Input: part model. Units: mm. Frame: model coordinates. Face numbers are marked on the shaded views. A direction names the side the tool comes from. Round coordinates to 2 decimals unless told otherwise and drop trailing zeros. Loops run counter-clockwise (first coordinate to the right, second up) from the corner with the lowest first, then second, coordinate; pieces in that order, holes last. Notation, with made-up numbers: M 19,57 L 27,57 A18 ccw 27,87 Z; hole C 60.5,34.5 d6. An arc over 180 degrees is marked long. Put each result on its own line as item: value. Start each with the question number.
1) Reachability of the marked faces 1 and 2 from +Z, -Z, +X, -X, +Y, -Y: full face, straight path, thin tool, end or side. Return the list, or none.
2) Section B-B on z = -25.5. Output: boundary loops of the cut face in (x, y) (3 decimals).
3) Line query: probe 1 along Y at (x, z) = (0, -151); probe 2 along Y at (x, z) = (0, -106) (3 decimals); probe 3 along Y at (x, z) = (0, -149). Output: solid intervals per line, ascending.
4) Section C-C on x = 0. State how many separate pieces and enclosed holes the cut face has, plus the area to 3 significant figures.
5) Draft query along X for the marked faces 3, 4, 5 and 6. Return one class per face: +X half, -X half, draft (parallel to the pull), parting line (faces both ways), or undercut.
6) Pin query (flat end, axial travel): pin 1 (2 mm diameter, centred on x = 6, z = -95, fed in from +Y); pin 2 (10.5 mm diameter, centred on x = 3.5, y = -2.5, fed in from +Z); pin 3 (16 mm diameter, centred on x = 4, y = 7, fed in from -Z). Return the tip coordinate at first contact, or that it passes through.
7) Section A-A on y = 0. Output: boundary loops of the cut face in (x, z) (3 decimals), plus the area to 3 significant figures.
from build123d import *
from OCP.BRepFilletAPI import BRepFilletAPI_MakeChamfer

# Parameters (mm, degrees)
CHAMFER1_SIZE           = 0.762
CHAMFER1_SIZE2          = 0.876580726
CUT_EXTRUDE1_DEPTH      = 193.922990854
CUT_EXTRUDE1_DEPTH_BACK = 193.922990854
SKETCH2_W               = 9.652
SKETCH2_H               = 20.7772
SKETCH3_R               = 3.9624
CUT_EXTRUDE2_DEPTH      = 193.922990854


with BuildPart() as part:
    # Sketch1 → Revolve1 (revolve)
    with BuildSketch(Plane(origin=(0, 0, 0), x_dir=(0, 0, -1), z_dir=(1, 0, 0)), mode=Mode.PRIVATE) as revolve1_sk:
        with BuildLine():
            Line((0, 8.7376), (0, 22.225))
            Line((0, 22.225), (127, 22.225))
            Line((127, 22.225), (141.697599691, 42.602209504))
            ThreePointArc((141.697599691, 42.602209504), (143.065361481, 51.010384281), (137.16, 57.15))
            Line((137.16, 57.15), (137.16, 76.2))
            Line((137.16, 76.2), (160.02, 76.2))
            Line((160.02, 76.2), (160.02, 57.15))
            Line((160.02, 57.15), (144.145832257, 35.141559942))
            ThreePointArc((144.145832257, 35.141559942), (142.376686305, 28.805838284), (145.135826502, 22.834373498))
            Line((145.135826502, 22.834373498), (152.0952, 15.875))
            Line((152.0952, 15.875), (152.0952, 8.7376))
            Line((152.0952, 8.7376), (0, 8.7376))
        make_face()
    revolve(revolve1_sk.sketch.rotate(Axis((0, 0, 0), (0, 0, -1)), 90), axis=Axis((0, 0, 0), (0, 0, -1)))

    # Chamfer1: one chamfer whose edges measure the first distance from different faces: ONE call of the kernel's chamfer builder (chamfer() names one face for all edges)
    chamfer1_edges_1 = [part.edges().sort_by_distance(p)[0] for p in [
        (-76.2, 0, -160.02),
    ]]
    chamfer1_side_1 = [part.faces().sort_by_distance(p)[0] for p in [
        (-74.044738531, 0, -160.02),
    ]]
    chamfer1_edges_2 = [part.edges().sort_by_distance(p)[0] for p in [
        (-76.2, 0, -137.16),
    ]]
    chamfer1_side_2 = [part.faces().sort_by_distance(p)[0] for p in [
        (-76.2, 0, -148.59),
    ]]
    chamfer1 = BRepFilletAPI_MakeChamfer(part.part.solid().wrapped)
    for e in chamfer1_edges_1:
        chamfer1.Add(CHAMFER1_SIZE, CHAMFER1_SIZE2, e.wrapped, chamfer1_side_1[0].wrapped)  # the first distance lies on this face
    for e in chamfer1_edges_2:
        chamfer1.Add(CHAMFER1_SIZE, CHAMFER1_SIZE2, e.wrapped, chamfer1_side_2[0].wrapped)  # the first distance lies on this face
    add(Compound.cast(chamfer1.Shape()), mode=Mode.REPLACE)

    # Sketch2 → Cut-Extrude1 (cut, two sides: drawn at the far end of the back side and taken through both)
    with BuildSketch(Plane(origin=(0, 0, 0), x_dir=(0, 0, -1), z_dir=(1, 0, 0)).offset(-CUT_EXTRUDE1_DEPTH_BACK)):
        with Locations((4.826, 0)):
            Rectangle(SKETCH2_W, SKETCH2_H)
    extrude(amount=CUT_EXTRUDE1_DEPTH + CUT_EXTRUDE1_DEPTH_BACK, mode=Mode.SUBTRACT)

    # Sketch3 → Cut-Extrude2 (cut, through all)
    with BuildSketch(Plane(origin=(0, 0, -160.02), x_dir=(-1, 0, 0), z_dir=(0, 0, -1))):
        with Locations((0, 66.675)):
            Circle(SKETCH3_R)
    extrude(amount=-CUT_EXTRUDE2_DEPTH, mode=Mode.SUBTRACT)


solid = part.part
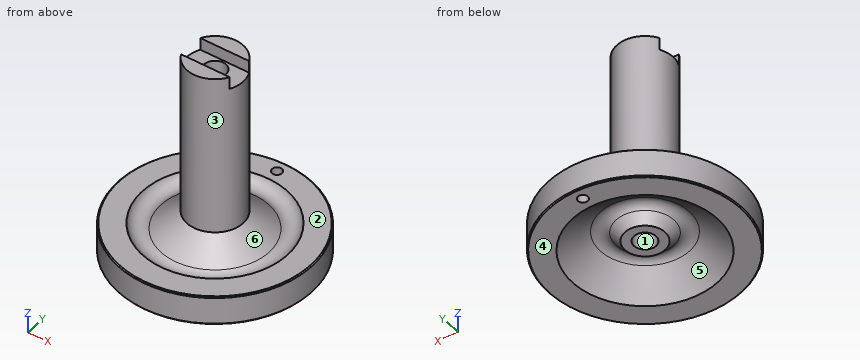
Geometry results:
1. face 1: +Z, -Z
1. face 2: +Z
2. outline: C 0,0 d44.45; hole C 0,0 d17.475
3. probe 1: y = -76.2 to -44.64, -16.97 to -8.74, 8.74 to 16.97, 44.64 to 62.71, 70.64 to 76.2
3. probe 2: y = -22.225 to -8.738, 8.738 to 22.225
3. probe 3: y = -76.2 to -41.87, -18.97 to -8.74, 8.74 to 18.97, 41.87 to 62.71, 70.64 to 76.2
4. separate pieces: 3
4. enclosed holes: 0
4. area: 5,500 mm²
5. face 3: parting line
5. face 4: draft
5. face 5: undercut
5. face 6: undercut
6. pin 1: stops at y = 21.66
6. pin 2: stops at z = -9.65
6. pin 3: stops at z = -152.1
7. outline: M -76.2,-159.143 L -75.438,-160.02 L -57.15,-160.02 L -35.142,-144.146 A9.525 cw -22.834,-145.136 L -15.875,-152.095 L -8.738,-152.095 L -8.738,-9.652 L -22.225,-9.652 L -22.225,-127 L -42.602,-141.698 A9.525 cw -57.15,-137.16 L -75.323,-137.16 L -76.2,-137.922 Z; M 8.738,-152.095 L 15.875,-152.095 L 22.834,-145.136 A9.525 cw 35.142,-144.146 L 57.15,-160.02 L 75.438,-160.02 L 76.2,-159.143 L 76.2,-137.922 L 75.323,-137.16 L 57.15,-137.16 A9.525 cw 42.602,-141.698 L 22.225,-127 L 22.225,-9.652 L 8.738,-9.652 Z
7. area: 5,450 mm²
